from build123d import *

# Parameters (mm, degrees)
F0_R     = 17.5
F1_DEPTH = 1.6
F0_R_2   = 19.1
F2_DEPTH = 6
F3_SIZE2 = 3
F3_SIZE  = 0.2
F4_R     = 2


with BuildPart() as f1:
    # F0 (on Top) → F1 (new body)
    with BuildSketch(Plane.XY):
        Circle(F0_R)
    extrude(amount=F1_DEPTH)

    # F0 (on Top) → F2 (join)
    with BuildSketch(Plane.XY):
        Circle(F0_R_2)
        Circle(F0_R, mode=Mode.SUBTRACT)
    extrude(amount=F2_DEPTH)

    # F3
    f3_edges = [f1.edges().sort_by_distance(p)[0] for p in [
        (-17.5, 0, 6),
    ]]
    chamfer(f3_edges, length=F3_SIZE, length2=F3_SIZE2)

    # F4
    f4_edges = [f1.edges().sort_by_distance(p)[0] for p in [
        (-19.1, 0, 0),
    ]]
    fillet(f4_edges, radius=F4_R)


solid = f1.part
Source: CAD feature listing. Evaluate the final solid. Frame: model axes, mm. A direction names the side the tool comes from. Round coordinates to 2 decimals unless told otherwise and drop trailing zeros. Loops run counter-clockwise (first coordinate to the right, second up) from the corner with the lowest first, then second, coordinate; pieces in that order, holes last.
Q1. Section A-A, the plane z = 4.65. Return loops of the section in (x, y).
Q2. Ray query, line 1 (Y direction, x = 0, z = 2.65); line 2 (Z direction, x = -11.5, y = -10); line 3 (Y direction, x = -5.5, z = 3.8). Return the intervals inside material, ascending.
Q3. Access query for faces 4 (the face through (6, -17, 6)), 5 (the face through (0, 0, 1.6)). Directions: +Z, -Z, +X, -X, +Y, -Y. A direction counts if a zero-diameter tool reaches every point of the face in a straight line with its end or side. Return the directions, or none.
Q4. Mould query, pull axis X, two halves, no side actions, for faces 1 (the face through (-15.16, -11.62, 3.97)), 2 (the face through (-13.9, -10.65, 3.15)), 3 (the face through (0, 0, 0)). Classes: pulls with the +X half, pulls with the -X half, needs draft (parallel to the pull), parting line crosses it, or undercut.
Q5. First-contact query: P1, Ø10.5, axis at x = 4.5, y = 7, coming from the +Z side; P2, Ø3, axis at x = -1.5, z = 1.5, coming from the +Y side; P3, Ø1, axis at x = -13, z = 3, coming from the +Y side. Flat tips, straight axial feed; report the tip coordinate or a pass-through.
Q6. Section B-B, the plane y = 0. Return loops of the section in (x, z).
Solutions:
1. outline: circle Ø38.2 at (0, 0); hole circle Ø35.22 at (0, 0)
2. line 1: y = -19.1 to -17.5, 17.5 to 19.1
2. line 2: z = 0 to 1.6
2. line 3: y = -18.29 to -16.67, 16.67 to 18.29
3. face 4: +Z, +X, -X, +Y, -Y
3. face 5: +Z
4. face 1: parting line crosses it
4. face 2: undercut
4. face 3: needs draft
5. P1: stops at z = 1.6
5. P2: stops at y = 19.1
5. P3: stops at y = 14.44
6. outline: (-19.1, 2) arc R2 ccw to (-17.1, 0) - (17.1, 0) arc R2 ccw to (19.1, 2) - (19.1, 6) - (17.7, 6) - (17.5, 3) - (17.5, 1.6) - (-17.5, 1.6) - (-17.5, 3) - (-17.7, 6) - (-19.1, 6) - close
